from build123d import *

# Parameters (mm, degrees)
F1_DEPTH = 3.175
F3_DEPTH = 12.7
F5_DEPTH = 25.4


with BuildPart() as f1:
    # F0 (on Top) → F1 (new body)
    with BuildSketch(Plane.XY):
        with BuildLine():
            Line((-58.565236, -28.575), (58.565236, -28.575))
            ThreePointArc((58.565236, -28.575), (57.770772, -21.846928), (63.5, -18.231118))
            Line((63.5, -18.231118), (63.5, 18.231118))
            ThreePointArc((63.5, 18.231118), (57.770772, 21.846928), (58.565236, 28.575))
            Line((58.565236, 28.575), (-58.565236, 28.575))
            ThreePointArc((-58.565236, 28.575), (-57.770772, 21.846928), (-63.5, 18.231118))
            Line((-63.5, 18.231118), (-63.5, -18.231118))
            ThreePointArc((-63.5, -18.231118), (-57.770772, -21.846928), (-58.565236, -28.575))
        make_face()
        with BuildLine():
            ThreePointArc((-54.012243, -25.4), (-55.495439, -19.421566), (-60.326977, -15.600862))
            Line((-60.326977, -15.600862), (-60.326977, 15.600862))
            ThreePointArc((-60.326977, 15.600862), (-55.495439, 19.421566), (-54.012243, 25.4))
            Line((-54.012243, 25.4), (54.012243, 25.4))
            ThreePointArc((54.012243, 25.4), (55.494871, 19.422448), (60.325, 15.601561))
            Line((60.325, 15.601561), (60.325, -15.601561))
            ThreePointArc((60.325, -15.601561), (55.494871, -19.422448), (54.012243, -25.4))
            Line((54.012243, -25.4), (-54.012243, -25.4))
        make_face(mode=Mode.SUBTRACT)
    extrude(amount=F1_DEPTH)

    # F2 (on face) → F3 (join)
    with BuildSketch(Plane(origin=(0, 0, 0), x_dir=(1, 0, 0), z_dir=(0, 0, -1))):
        with BuildLine():
            ThreePointArc((55.955421, -27.0002), (56.664977, -20.573888), (61.9252, -16.814766))
            Line((61.9252, -16.814766), (61.9252, 16.814766))
            ThreePointArc((61.9252, 16.814766), (56.664977, 20.573888), (55.955421, 27.0002))
            Line((55.955421, 27.0002), (-55.955421, 27.0002))
            ThreePointArc((-55.955421, 27.0002), (-56.665487, 20.573018), (-61.927177, 16.814364))
            Line((-61.927177, 16.814364), (-61.927177, -16.814364))
            ThreePointArc((-61.927177, -16.814364), (-56.665487, -20.573018), (-55.955421, -27.0002))
            Line((-55.955421, -27.0002), (55.955421, -27.0002))
        make_face()
        with BuildLine():
            Line((-54.012243, 25.4), (54.012243, 25.4))
            ThreePointArc((54.012243, 25.4), (55.494871, 19.422448), (60.325, 15.601561))
            Line((60.325, 15.601561), (60.325, -15.601561))
            ThreePointArc((60.325, -15.601561), (55.494871, -19.422448), (54.012243, -25.4))
            Line((54.012243, -25.4), (-54.012243, -25.4))
            ThreePointArc((-54.012243, -25.4), (-55.495439, -19.421566), (-60.326977, -15.600862))
            Line((-60.326977, -15.600862), (-60.326977, 15.600862))
            ThreePointArc((-60.326977, 15.600862), (-55.495439, 19.421566), (-54.012243, 25.4))
        make_face(mode=Mode.SUBTRACT)
    extrude(amount=F3_DEPTH)

    # F4 (on face) → F5 (cut)
    with BuildSketch(Plane.XY.offset(3.175)):
        with BuildLine():
            ThreePointArc((-55.926105, 25.4), (-56.876639, 20.816906), (-60.326977, 17.654086))
            Line((-60.326977, 17.654086), (-60.326977, 16.823715))
            ThreePointArc((-60.326977, 16.823715), (-56.322288, 20.255613), (-55.160073, 25.4))
            Line((-55.160073, 25.4), (-55.926105, 25.4))
        make_face()
        with BuildLine():
            ThreePointArc((55.160073, 25.4), (56.322288, 20.255613), (60.326977, 16.823715))
            Line((60.326977, 16.823715), (60.326977, 17.654086))
            ThreePointArc((60.326977, 17.654086), (56.876639, 20.816906), (55.926105, 25.4))
            Line((55.926105, 25.4), (55.160073, 25.4))
        make_face()
        with BuildLine():
            ThreePointArc((-55.160073, -25.4), (-56.322288, -20.255613), (-60.326977, -16.823715))
            Line((-60.326977, -16.823715), (-60.326977, -17.654086))
            ThreePointArc((-60.326977, -17.654086), (-56.876639, -20.816906), (-55.926105, -25.4))
            Line((-55.926105, -25.4), (-55.160073, -25.4))
        make_face()
        with BuildLine():
            Line((60.326977, -17.654086), (60.326977, -16.823715))
            ThreePointArc((60.326977, -16.823715), (56.322288, -20.255613), (55.160073, -25.4))
            Line((55.160073, -25.4), (55.926105, -25.4))
            ThreePointArc((55.926105, -25.4), (56.876639, -20.816906), (60.326977, -17.654086))
        make_face()
    extrude(amount=-F5_DEPTH, mode=Mode.SUBTRACT)


solid = f1.part
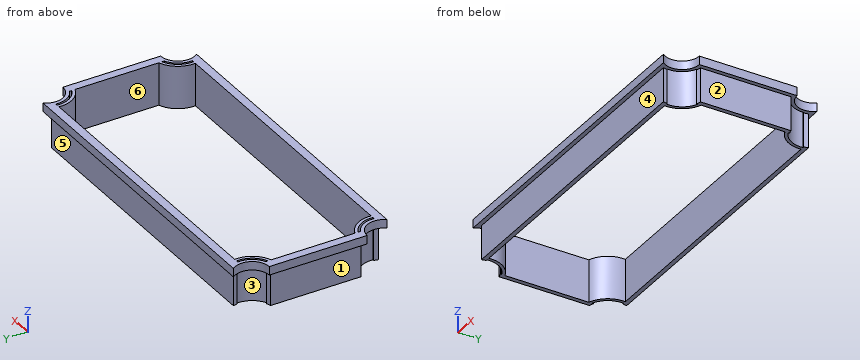
Can you work these out from the model? Positions are in its coordinate system, mm. Face numbers are marked on the shaded views. A direction names the side the tool comes from. Coordinates: 2 decimals unless noted, no trailing zeros. Write each loop counter-clockwise with the first axis right and the second up, starting at its lowest first coordinate (ties: lowest second). Pieces come first, ordered by that corner, then holes. Notation, with made-up numbers: (-4, 31.25) - (7, 31.25) arc R12 cw to (7, 35.25) - close; hole circle Ø10 at (0.25, -8). An arc over 180 degrees is marked (long way). Return JSON: item names as keys, results as strings. Group by question number.
Item 1: If we section it at D-D (y = 24): Write out the boundary of the cut face in (x, z) (3 decimals).
Item 2: If we section it at A-A (x = -26): Write out the boundary of the cut face in (y, z) (3 decimals).
Item 3: Please list where these lines run through material, in increasing order: probe 1 along X at (y, z) = (13.5, 0.25) (3 decimals); probe 2 along Y at (x, z) = (19, -2.75); probe 3 along X at (y, z) = (-9, -6.25) (3 decimals).
Item 4: We'd pull the mould along X, two halves only. Please class the marked faces 1, 2, 3 and 4: pulls with the +X half, pulls with the -X half, needs draft (parallel to the pull), parting line crosses it, or undercut.
Item 5: If we section it at B-B (y = -6): Write out the boundary of the cut face in (x, z) (3 decimals).
Item 6: I'm going to push flat-ended pins straight in: pin 1 Ø0.8 at (x, z) = (-55.5, -3) entering from +Y; pin 2 Ø6 at (x, z) = (-16, -2) entering from +Y (3 decimals); pin 3 Ø1 at (y, z) = (-11, -5.5) entering from -X; pin 4 Ø6.5 at (x, z) = (13.5, -3.5) entering from -Y. Where does each tip first touch, or does it pass through?
Item 7: Which directions (+Z, -Z, +X, -X, +Y, -Y) give clear straight access to the entire face, cutting with the end or side of a thin tool? Please do the marked faces 5 and 6.
Return value:
{
 "1": {"outline": "(-57.179, 0) - (-55.904, 0) - (-55.904, 3.175) - (-57.179, 3.175) - close; (-55.14, -12.7) - (-53.995, -12.7) - (-53.995, 3.175) - (-55.14, 3.175) - close; (53.995, -12.7) - (55.14, -12.7) - (55.14, 3.175) - (53.995, 3.175) - close; (55.904, 0) - (57.179, 0) - (57.179, 3.175) - (55.904, 3.175) - close"},
 "2": {"outline": "(-28.575, 0) - (-27, 0) - (-27, -12.7) - (-25.4, -12.7) - (-25.4, 3.175) - (-28.575, 3.175) - close; (25.4, -12.7) - (27, -12.7) - (27, 0) - (28.575, 0) - (28.575, 3.175) - (25.4, 3.175) - close"},
 "3": {"probe 1": "x = -63.5 to -60.327, 60.325 to 63.5", "probe 2": "y = -27 to -25.4, 25.4 to 27", "probe 3": "x = -61.927 to -60.327, 60.325 to 61.925"},
 "4": {"face 1": "pulls with the -X half", "face 2": "pulls with the +X half", "face 3": "undercut", "face 4": "needs draft"},
 "5": {"outline": "(-63.5, 0) - (-61.927, 0) - (-61.927, -12.7) - (-60.327, -12.7) - (-60.327, 3.175) - (-63.5, 3.175) - close; (60.325, -12.7) - (61.925, -12.7) - (61.925, 0) - (63.5, 0) - (63.5, 3.175) - (60.325, 3.175) - close"},
 "6": {"pin 1": "stops at y = 27", "pin 2": "stops at y = 28.575", "pin 3": "stops at x = -61.93", "pin 4": "stops at y = -27"},
 "7": {"face 5": "-Z, +X, -X, +Y", "face 6": "+Z, -Z"}
}
